Verification items for the finished model (mm, model axes). Face numbers are marked on the shaded views. A direction names the side the tool comes from. Give positions to 0.01 mm unless a question says otherwise; leave off trailing zeros. Order: outer loops, then holes, each group sorted by start corner. A loop starts at its lowest first (then second) coordinate and runs counter-clockwise, first axis right, second up. Notation, with made-up numbers: (47.25, -33.5) -> (66.25, -33.5) arc R17 ccw to (66.25, -29.5) -> close; hole circle Ø9 at (35, 4.5). An arc over 180 degrees is marked (long way). Write each question's results on one line, items separated by ' | '. Start each with the question number.
1. Cross-section at B-B, the plane x = -14. Enter the section's corners in (y, z).
2. Cross-section at C-C, the plane y = -67.5. Enter the section's corners in (x, z), then the cut area to 3 significant figures.
3. Depth check by flat-ended pin: pin 1 Ø12 at (x, z) = (-42, 8.5) entering from +Y; pin 2 Ø12 at (y, z) = (-64.5, -2) entering from -X; pin 3 Ø10 at (y, z) = (-12, -11.5) entering from -X; pin 4 Ø8.5 at (x, y) = (10, 60) entering from -Z. Enter the tip coordinate at first touch or a pass-through.
4. Set-up check for the marked faces 1, 2 and 3: record each of +Z, -Z, +X, -X, +Y, -Y from which the full face is reachable in a straight line by a thin tool's end or side.
5. Mould release check, pull along Y, two halves, no side actions. Record for the marked faces 4, 5 and 6: +Y half, -Y half, draft (parallel to the pull), parting line (faces both ways), or undercut.
6. Material ranges on L1, parallel to X at y = -46, z = 13; L2, parallel to X at y = -34.5, z = -16; L3, parallel to Y at x = -12.5, z = -6.5, recorded low to high. Write a range as from..to.
7. Cross-section at A-A, the plane y = 21.5. Enter the section's corners in (x, z).
8. Cross-section at D-D, the plane z = -7. State how many separate pieces and enclosed holes the cut face has, then the cut area to 3 significant figures.
from build123d import *

# Parameters (mm, degrees)
BOSS_EXTRUDE1_DEPTH      = 20
BOSS_EXTRUDE1_DEPTH_BACK = 20
SKETCH1_R                = 7
SKETCH2_W                = 100
SKETCH2_H                = 10
BOSS_EXTRUDE2_DEPTH      = 40
FILLET1_R                = 20
SKETCH3_R                = 10
CUT_EXTRUDE1_DEPTH       = 40
FILLET2_SIZE             = 10
SKETCH4_W                = 20
SKETCH4_H                = 70
CUT_EXTRUDE2_DEPTH       = 50
SKETCH5_R                = 15
BOSS_EXTRUDE3_DEPTH      = 10
CUT_EXTRUDE4_DEPTH       = 10
CUT_EXTRUDE4_DEPTH_BACK  = 56


# Some blends are built 0.0001 mm under size
with BuildPart() as part:
    # Sketch1 → Boss-Extrude1 (new, two sides: drawn at the far end of the back side and taken through both)
    with BuildSketch(Plane.XY.offset(-BOSS_EXTRUDE1_DEPTH_BACK)):
        with BuildLine():
            Line((0, 0), (0, 60))
            ThreePointArc((0, 60), (8.220336618, 69.840365758), (19.36655965, 63.502507721))
            Line((19.36655965, 63.502507721), (35, 0))
            Line((35, 0), (35, -110))
            Line((35, -110), (0, -110))
            Line((0, -110), (0, -90))
            Line((0, -90), (0, -20))
            Line((0, -20), (-42, -20))
            Line((-42, -20), (-42, 0))
            Line((-42, 0), (0, 0))
        make_face()
        with Locations((10, 60)):
            Circle(SKETCH1_R, mode=Mode.SUBTRACT)
    extrude(amount=BOSS_EXTRUDE1_DEPTH + BOSS_EXTRUDE1_DEPTH_BACK)

    # Sketch2 → Boss-Extrude2 (add)
    with BuildSketch(Plane.XY.offset(20)):
        with Locations((-15, -105)):
            Rectangle(SKETCH2_W, SKETCH2_H)
    extrude(amount=-BOSS_EXTRUDE2_DEPTH)

    # Fillet1
    fillet1_edges = [part.edges().sort_by_distance(p)[0] for p in [
        (-42, -10, 20),
        (-42, -10, -20),
    ]]
    fillet(fillet1_edges, radius=FILLET1_R - 0.0001)  # a hair under: the kernel refuses the full size

    # Sketch3 → Cut-Extrude1 (cut)
    with BuildSketch(Plane(origin=(0, 0, 0), x_dir=(1, 0, 0), z_dir=(0, 1, 0))):
        with Locations(Location((-22, 0, 0), (0, 0, 270))):
            Circle(SKETCH3_R)
    extrude(amount=-CUT_EXTRUDE1_DEPTH, mode=Mode.SUBTRACT)

    # Fillet2
    # a fillet whose section is not a circle: 10 mm, written as the material it adds along each edge
    with BuildSketch(Plane(origin=(0, -20, 20), x_dir=(-1, 0, 0), z_dir=(0, 0, -1))) as fillet2_piece_1:
        with BuildLine():
            add(Edge.make_bspline([(FILLET2_SIZE, 0), (FILLET2_SIZE * 0.831801948466, 0), (FILLET2_SIZE * 0.663603896932, 0), (FILLET2_SIZE * 0.292893218813, -FILLET2_SIZE * 0.0716919198361), (FILLET2_SIZE * 0.0716919198361, -FILLET2_SIZE * 0.292893218813), (0, -FILLET2_SIZE * 0.663603896932), (0, -FILLET2_SIZE * 0.831801948466), (0, -FILLET2_SIZE)], knots=[0, 0, 0, 0, 0, 0, 0.5, 0.5, 1, 1, 1, 1, 1, 1], degree=5))
            Line((0, -FILLET2_SIZE), (-FILLET2_SIZE * 0.02, -FILLET2_SIZE))
            Line((-FILLET2_SIZE * 0.02, -FILLET2_SIZE), (-FILLET2_SIZE * 0.02, FILLET2_SIZE * 0.02))
            Line((-FILLET2_SIZE * 0.02, FILLET2_SIZE * 0.02), (FILLET2_SIZE, FILLET2_SIZE * 0.02))
            Line((FILLET2_SIZE, FILLET2_SIZE * 0.02), (FILLET2_SIZE, 0))
        make_face()
    extrude(amount=40)

    # Sketch4 → Cut-Extrude2 (cut)
    with BuildSketch(Plane.ZY):
        with Locations((0, 35)):
            Rectangle(SKETCH4_W, SKETCH4_H)
    extrude(amount=-CUT_EXTRUDE2_DEPTH, mode=Mode.SUBTRACT)

    # Sketch5 → Boss-Extrude3 (add)
    with BuildSketch(Plane(origin=(0, -100, 0), x_dir=(1, 0, 0), z_dir=(0, 1, 0))):
        with Locations(Location((-22, 0, 0), (0, 0, 180))):
            Circle(SKETCH5_R)
    extrude(amount=BOSS_EXTRUDE3_DEPTH)

    # Sketch6 → Cut-Extrude4 (cut, two sides: drawn at the far end of the back side and taken through both)
    with BuildSketch(Plane.XY.offset(20).offset(-CUT_EXTRUDE4_DEPTH_BACK)):
        Polygon((30, -47.923364513), (30, -7.018043607), (7.243954377, -27.498484668), align=None)
        Polygon((27.757729325, -5), (5, -5), (5, -25.481956393), align=None)
        Polygon((27.736463224, -49.922898925), (5, -29.515595427), (5, -30), (5, -75.254357341), align=None)
        Polygon((30, -97.981956393), (30, -51.892301788), (7.116883504, -77.387151546), align=None)
        Polygon((27.757729325, -100), (5, -79.518043607), (5, -100), align=None)
        with BuildLine():
            Line((29.850709662, 0), (17.404345208, 50.556712859))
            ThreePointArc((17.404345208, 50.556712859), (11.407865959, 48.082873105), (5, 49.091287885))
            Line((5, 49.091287885), (5, 0))
            Line((5, 0), (29.850709662, 0))
        make_face()
    extrude(amount=CUT_EXTRUDE4_DEPTH + CUT_EXTRUDE4_DEPTH_BACK, mode=Mode.SUBTRACT)


solid = part.part
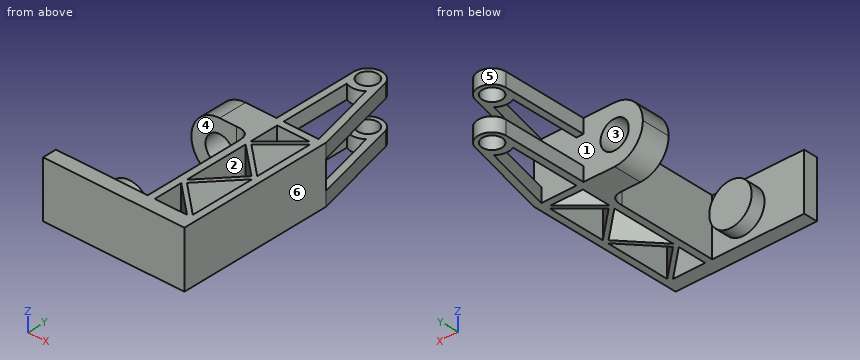
Results below:
1) outline: (-110, -20) -> (-100, -20) -> (-100, -12.69) -> (-90, -12.69) -> (-90, 12.69) -> (-100, 12.69) -> (-100, 20) -> (-110, 20) -> close; (-20, -20) -> (0, -20) -> (0, -6) -> (-20, -6) -> close; (-20, 6) -> (0, 6) -> (0, 20) -> (-20, 20) -> close
2) outline: (0, -20) -> (5, -20) -> (5, 20) -> (0, 20) -> close; (11.96, -20) -> (15.99, -20) -> (15.99, 20) -> (11.96, 20) -> close; (30, -20) -> (35, -20) -> (35, 20) -> (30, 20) -> close | area: 561 mm²
3) pin 1: stops at y = 0 | pin 2: stops at x = 0 | pin 3: stops at x = -40.91 | pin 4: passes through
4) face 1: none | face 2: +Z, -Z | face 3: +Y
5) face 4: undercut | face 5: +Y half | face 6: draft
6) L1: x = 0..5, 23.37..27.86, 30..35 | L2: x = 0..5, 10.55..15.04, 30..35 | L3: y = -110..-90, -20..0
7) outline: (0, -20) -> (5, -20) -> (5, -10) -> (0, -10) -> close; (0, 10) -> (5, 10) -> (5, 20) -> (0, 20) -> close; (24.56, -20) -> (29.71, -20) -> (29.71, -10) -> (24.56, -10) -> close; (24.56, 10) -> (29.71, 10) -> (29.71, 20) -> (24.56, 20) -> close
8) separate pieces: 2 | enclosed holes: 5 | area: 3,330 mm²
